The model under review builds one solid part; all positions refer to its coordinate system, in mm. A direction names the side the tool comes from. Round coordinates to 2 decimals unless told otherwise and drop trailing zeros. Write each loop counter-clockwise with the first axis right and the second up, starting at its lowest first coordinate (ties: lowest second). Pieces come first, ordered by that corner, then holes.
Item 1: Draft analysis for pull direction X (two halves, no side actions). For faces 5 (the face through (-7.5, 25, 21)), 6 (the face through (-6.55, 25, 5)), 7 (the face through (-0.165, 33.045, 46.63)), state which applies: +X half, -X half, draft (parallel to the pull), parting line (faces both ways), or undercut.
Item 2: Clearance check with flat-ended pins moving along their axes: pin 1 Ø1.5 at (y, z) = (31, 8.5) entering from -X; pin 2 Ø0.8 at (x, z) = (-2, 34.5) entering from -Y; pin 3 Ø1 at (x, y) = (-0.5, 30.5) entering from -Z; pin 4 Ø3 at (x, y) = (6, 33) entering from -Z. State where each tip first meets the part, or that it passes through.
Item 3: Add section A-A (x = 5). Give the boundary of the cut face in (y, z).
Item 4: To check wall thickness, follow L1, parallel to Z at x = 4.5, y = 28.25; L2, parallel to Z at x = 3.75, y = 27; L3, parallel to Y at x = 5, z = 22.5. State the ranges of each line that lie inside material, in increasing order.
Item 5: Add section B-B (z = 8.5). Give the boundary of the cut face in (x, y), plus the area to 3 significant figures.
Item 6: Machinability: for faces 1 (the face through (-0.105, 27.683, 33.692)), 2 (the face through (0.105, 20.856, 10.825)), 3 (the face through (-4.97, 24.74, 7.55)), 4 (the face through (0.1, 31.1, 41.1)), which of the approach directions +Z, -Z, +X, -X, +Y, -Y give a long, thin tool a straight path to every point of the face, cutting with its end or side? Answer none if there is none.
Item 7: Add section C-C (x = -5.25). Give the boundary of the cut face in (y, z).
Item 8: Add section D-D (z = 26). Give the boundary of the cut face in (x, y), plus the area to 3 significant figures.
```python
from build123d import *

# Parameters (mm, degrees)
SKETCH_10_W         = 15
SKETCH_10_H         = 8
EXTRUDE_7_DEPTH     = 26
CUT_EXTRUDE_4_DEPTH = 11
SKETCH_12_W         = 15
SKETCH_12_H         = 6
EXTRUDE_8_DEPTH     = 6
SKETCH_14_W         = 15
SKETCH_14_H         = 5
EXTRUDE_9_DEPTH     = 4
EXTRUDE_10_DEPTH    = 15
EXTRUDE_11_DEPTH    = 5
SKETCH_19_R         = 1.1
CUT_EXTRUDE_5_DEPTH = 5
EXTRUDE_START       = 0.5
SKETCH_20_R         = 1.5
SKETCH_20_R_2       = 1.1
EXTRUDE_12_DEPTH    = 0.5
SKETCH_21_R         = 1.5
SKETCH_21_R_2       = 1.1
EXTRUDE_13_DEPTH    = 0.5
FILLET_4_R          = 0.5
CHAMFER_1_SIZE      = 4.493554602
CHAMFER_1_SIZE_2    = 2.7
FILLET_7_R          = 2
SKETCH_22_W         = 15
SKETCH_22_H         = 2
CUT_EXTRUDE_6_DEPTH = 15
FILLET_8_R          = 10
FILLET_9_R          = 5
FILLET_10_R         = 2


# Some blends are built 0.0001 mm under size
with BuildPart() as part:
    # 草图10 → 凸台-拉伸7 (new body)
    with BuildSketch(Plane.XY):
        with Locations((0, 24.68211788)):
            Rectangle(SKETCH_10_W, SKETCH_10_H)
    extrude(amount=EXTRUDE_7_DEPTH)

    # 草图11 → 切除-拉伸4 (cut)
    with BuildSketch(Plane(origin=(0, 28.68211788, 0), x_dir=(1, 0, 0), z_dir=(0, 1, 0))):
        with BuildLine():
            Line((-3.45, -4), (-3.45, -6))
            ThreePointArc((-3.45, -6), (-5, -7.55), (-6.55, -6))
            Line((-6.55, -6), (-6.55, -4))
            ThreePointArc((-6.55, -4), (-5, -2.45), (-3.45, -4))
        make_face()
        with BuildLine():
            Line((3.45, -4), (3.45, -6))
            ThreePointArc((3.45, -6), (5, -7.55), (6.55, -6))
            Line((6.55, -6), (6.55, -4))
            ThreePointArc((6.55, -4), (5, -2.45), (3.45, -4))
        make_face()
    extrude(amount=-CUT_EXTRUDE_4_DEPTH, mode=Mode.SUBTRACT)

    # 草图12 → 凸台-拉伸8 (add)
    with BuildSketch(Plane.XY.offset(26)):
        with Locations((0, 25.68211788)):
            Rectangle(SKETCH_12_W, SKETCH_12_H)
    extrude(amount=EXTRUDE_8_DEPTH)

    # 草图14 → 凸台-拉伸9 (add)
    with BuildSketch(Plane.XY.offset(32)):
        with Locations((0, 23.5)):
            Rectangle(SKETCH_14_W, SKETCH_14_H)
    extrude(amount=EXTRUDE_9_DEPTH)

    # 草图17 → 凸台-拉伸10 (add)
    with BuildSketch(Plane.ZY.offset(7.5)):
        Polygon((36, 26), (39.535533906, 29.535533906), (43.071067812, 26), (38.071067812, 21), (36, 21), align=None)
    extrude(amount=-EXTRUDE_10_DEPTH)

    # 草图18 → 凸台-拉伸11 (add)
    with BuildSketch(Plane(origin=(0, -8.535533906, 8.535533906), x_dir=(1, 0, 0), z_dir=(0, -0.7071067811865507, 0.7071067811865445))):
        with BuildLine():
            Line((7.5, 48.840620434), (-7.5, 48.840620434))
            ThreePointArc((-7.5, 48.840620434), (0, 56.340620434), (7.5, 48.840620434))
        make_face()
    extrude(amount=-EXTRUDE_11_DEPTH)

    # 草图19 → 切除-拉伸5 (cut)
    with BuildSketch(Plane(origin=(0, -8.535533906, 8.535533906), x_dir=(1, 0, 0), z_dir=(0, -0.7071067811865507, 0.7071067811865445))):
        with Locations(Location((0, 48.840620434, 0), (0, 0, 270))):
            Circle(SKETCH_19_R)
    extrude(amount=-CUT_EXTRUDE_5_DEPTH, mode=Mode.SUBTRACT)

    # 草图20 → 凸台-拉伸12 (add)
    with BuildSketch(Plane(origin=(0, -8.535533906, 8.535533906), x_dir=(1, 0, 0), z_dir=(0, -0.7071067811865507, 0.7071067811865445)).offset(EXTRUDE_START)):
        with Locations(Location((0, 48.840620434, 0), (0, 0, 270))):
            Circle(SKETCH_20_R)
        with Locations(Location((0, 48.840620434, 0), (0, 0, 270))):
            Circle(SKETCH_20_R_2, mode=Mode.SUBTRACT)
    extrude(amount=-EXTRUDE_12_DEPTH)

    # 草图21 → 凸台-拉伸13 (add)
    with BuildSketch(Plane(origin=(0, -5, 5), x_dir=(1, 0, 0), z_dir=(0, 0.7071067811865513, -0.7071067811865437))):
        with Locations(Location((0, -48.840620434, 0), (0, 0, 90))):
            Circle(SKETCH_21_R)
        with Locations(Location((0, -48.840620434, 0), (0, 0, 90))):
            Circle(SKETCH_21_R_2, mode=Mode.SUBTRACT)
    extrude(amount=EXTRUDE_13_DEPTH)

    # 圆角4
    fillet_4_edges = [part.edges().sort_by_distance(p)[0] for p in [
        (0, 27.060660172, 44.131727984),
        (0, 30.596194078, 40.596194078),
    ]]
    fillet(fillet_4_edges, radius=FILLET_4_R - 0.0001)  # a hair under: the kernel refuses the full size

    # 倒角1
    # the kernel refuses this chamfer: 4.493554602, 2.7 mm, written as the material it adds along each edge
    with BuildSketch(Plane(origin=(-7.5, 26, 32), x_dir=(0, -0.019914630580833353, 0.9998016840798123), z_dir=(1, 0, 0))) as chamfer_1_piece_1_section:
        Polygon((CHAMFER_1_SIZE * 0.999801684157, -CHAMFER_1_SIZE * 0.0199146305824), (-CHAMFER_1_SIZE_2 * 0.0199146305808, -CHAMFER_1_SIZE_2 * 0.99980168408), (0, 0), align=None)
    chamfer_1_piece_1 = extrude(amount=15, mode=Mode.PRIVATE)
    chamfer_1_piece_1 = split(chamfer_1_piece_1, bisect_by=Plane(origin=(0, 28.68211788, 33.477199106), z_dir=(0, -1, 0)), keep=Keep.TOP, mode=Mode.PRIVATE)
    add(chamfer_1_piece_1)

    # 圆角7
    fillet_7_edges = [part.edges().sort_by_distance(p)[0] for p in [
        (0, 26.18524881, 36.18524881),
        (0, 28.68211788, 32.029760846),
    ]]
    fillet(fillet_7_edges, radius=FILLET_7_R)

    # 草图22 → 切除-拉伸6 (cut)
    with BuildSketch(Plane.XY.offset(26)):
        with Locations((0, 21.68211788)):
            Rectangle(SKETCH_22_W, SKETCH_22_H)
    extrude(amount=-CUT_EXTRUDE_6_DEPTH, mode=Mode.SUBTRACT)

    # 圆角8
    # the kernel refuses this fillet: 10 mm, written as the material it adds along each edge
    with BuildSketch(Plane(origin=(7.5, 22.68211788, 11), x_dir=(0, -1, 0), z_dir=(-1, 0, 0))) as fillet_8_piece_1:
        with BuildLine():
            CenterArc((10, 6), FILLET_8_R, 180, 36.869897646)
            Line((0, 6), (-0.2, 6))
            Line((-0.2, 6), (-0.2, 0))
            Line((-0.2, 0), (0, -0.2))
            ThreePointArc((0, -0.2), (1, -0.2), (1.84, -0.12))
            Line((1.84, -0.12), (2, 0))
        make_face()
    extrude(amount=15)
    with BuildSketch(Plane(origin=(7.5, 22.68211788, 32), x_dir=(0, 0, -1), z_dir=(-1, 0, 0))) as fillet_8_piece_2:
        with BuildLine():
            CenterArc((5.550931186, 10), FILLET_8_R, 236.282871199, 33.717128801)
            Line((0, 1.68211788), (-0.111018624, 1.515760238))
            ThreePointArc((-0.111018624, 1.515760238), (-0.2, 0.84105894), (-0.2, 0))
            Line((-0.2, 0), (0, -0.2))
            Line((0, -0.2), (5.550931186, -0.2))
            Line((5.550931186, -0.2), (5.550931186, 0))
        make_face()
    extrude(amount=15)

    # 圆角9
    fillet_9_edges = [part.edges().sort_by_distance(p)[0] for p in [
        (0, 20.68211788, 11),
        (0, 21, 32),
        (0, 21, 38.071067812),
    ]]
    fillet(fillet_9_edges, radius=FILLET_9_R)

    # 圆角10
    fillet_10_edges = [part.edges().sort_by_distance(p)[0] for p in [
        (0, 28.68211788, 0),
    ]]
    fillet(fillet_10_edges, radius=FILLET_10_R)


solid = part.part
```
Numbers:
1. face 5: -X half
1. face 6: undercut
1. face 7: parting line
2. pin 1: passes through
2. pin 2: stops at y = 21
2. pin 3: stops at z = 39.57
2. pin 4: stops at z = 41.5
3. outline: (20.68, 0) - (26.68, 0) arc R2 ccw to (28.68, 2) - (28.68, 2.45) - (20.68, 2.45) - close; (20.68, 7.55) - (28.68, 7.55) - (28.68, 31.48) arc R2 ccw to (28.4, 32.51) - (26.99, 34.85) arc R2 cw to (27.29, 37.29) - (33.49, 43.49) - (29.95, 47.02) - (22.46, 39.54) arc R5 ccw to (21, 36) - (21, 33.35) arc R5 ccw to (21.56, 31.05) arc R10 cw to (22.68, 26.45) - (22.68, 17) arc R10 cw to (21.35, 12.01) arc R5 ccw to (20.68, 9.52) - close
4. L1: z = 0.76 to 2.53, 7.47 to 32.75, 38.25 to 45.32
4. L2: z = 0.03 to 3.08, 6.92 to 34.83, 36.92 to 44.07
4. L3: y = 22.68 to 28.68
5. outline: (-7.5, 20.68) - (7.5, 20.68) - (7.5, 28.68) - (-7.5, 28.68) - close
5. area: 120 mm2
6. face 1: +X, -X, +Y
6. face 2: +X, -X, -Y
6. face 3: +Y, -Y
6. face 4: +Y
7. outline: (20.68, 0) - (26.68, 0) arc R2 ccw to (28.68, 2) - (28.68, 2.47) - (20.68, 2.47) - close; (20.68, 7.53) - (28.68, 7.53) - (28.68, 31.48) arc R2 ccw to (28.4, 32.51) - (26.99, 34.85) arc R2 cw to (27.29, 37.29) - (33.32, 43.32) - (29.79, 46.86) - (22.46, 39.54) arc R5 ccw to (21, 36) - (21, 33.35) arc R5 ccw to (21.56, 31.05) arc R10 cw to (22.68, 26.45) - (22.68, 17) arc R10 cw to (21.35, 12.01) arc R5 ccw to (20.68, 9.52) - close
8. outline: (-7.5, 22.68) - (7.5, 22.68) - (7.5, 28.68) - (-7.5, 28.68) - close
8. area: 90.0 mm2
